```python
from build123d import *

# Parameters (mm, degrees)
F1_DEPTH = 40.7
F2_R     = 4
F3_DEPTH = 25


with BuildPart() as f1:
    # F0 (on Front) → F1 (new body)
    with BuildSketch(Plane.XZ):
        Polygon((7.9, 80), (0, 80), (0, 3), (3, 0), (80, 0), (80, 7.9), (7.9, 7.9), align=None)
    extrude(amount=F1_DEPTH)

    # F2 (on face) → F3 (cut)
    with BuildSketch(Plane.YZ.offset(7.9)):
        with Locations((-31.2, 59.8)):
            Circle(F2_R)
        with Locations((-31.2, 46.8)):
            Circle(F2_R)
        with Locations((-10.5, 46.8)):
            Circle(F2_R)
        with Locations((-10.5, 59.8)):
            Circle(F2_R)
    extrude(amount=-F3_DEPTH, mode=Mode.SUBTRACT)


solid = f1.part
```
Could you check a few things on this model? Use its own coordinates, in mm. A direction names the side the tool comes from. Round coordinates to 2 decimals unless told otherwise and drop trailing zeros. Loops run counter-clockwise (first coordinate to the right, second up) from the corner with the lowest first, then second, coordinate; pieces in that order, holes last. Notation, with made-up numbers: (52.5, -14.75) - (72.5, -14.75) arc R29 cw to (72.5, 12.25) - close; hole circle Ø7 at (35, -18). An arc over 180 degrees is marked (long way). Answer in a Markdown table with one row per item. Add a question column.
(1) I need wall thicknesses on line 1 along Z through (x, y) = (3.25, -31.2); line 2 along Y through (x, z) = (2, 46); line 3 along Z through (x, y) = (2, -31) (3 decimals). Which ranges of each line are inside material? Lowest first, please.
(2) If we section it at C-C (y = -16): Please give me the cut outline in (x, z).
(3) For faces 5 (the face through (0, -20, 42)), 6 (the face through (44, -20, 7.9)), which set-ups out of +Z, -Z, +X, -X, +Y, -Y let a thin tool reach every point of the face, with its end or its side?
(4) If we section it at B-B (z = 46.8): Please give me the cut outline in (x, y).
(5) If we mould it in two halves opening along Z, with no side actions, what happens to faces 1 (the face through (41, -20, 0)), 2 (the face through (7.9, -20, 43)), 3 (the face through (4.005, -11.367, 55.895)), 4 (the face through (4.005, -27.505, 58.268))? For each: pulls with the +Z half, pulls with the -Z half, needs draft (parallel to the pull), parting line crosses it, or undercut.
(6) If we section it at A-A (y = -31.2): Please give me the cut outline in (x, z).
(7) I'm going to push flat-ended pins straight in: pin 1 (8 mm diameter, centred on x = 23.5, y = -15.5, fed in from +Z); pin 2 (10.5 mm diameter, centred on y = -10.5, z = 59.8, fed in from -X); pin 3 (13 mm diameter, centred on y = -10.5, z = 46.8, fed in from +X). Where does each tip first touch, or does it pass through?
(8) If we section it at D-D (z = 62): Please give me the cut outline in (x, y).
Model answer:
| question | item | result |
|---|---|---|
| 1 | line 1 | z = 0 to 42.8, 50.8 to 55.8, 63.8 to 80 |
| 1 | line 2 | y = -40.7 to -35.12, -27.28 to -14.42, -6.58 to 0 |
| 1 | line 3 | z = 1 to 42.805, 50.795 to 55.805, 63.795 to 80 |
| 2 | outline | (0, 3) - (3, 0) - (80, 0) - (80, 7.9) - (7.9, 7.9) - (7.9, 80) - (0, 80) - close |
| 3 | face 5 | +Z, -Z, -X, +Y, -Y |
| 3 | face 6 | +Z, +X, +Y, -Y |
| 4 | outline | (0, -40.7) - (7.9, -40.7) - (7.9, -35.2) - (0, -35.2) - close; (0, -27.2) - (7.9, -27.2) - (7.9, -14.5) - (0, -14.5) - close; (0, -6.5) - (7.9, -6.5) - (7.9, 0) - (0, 0) - close |
| 5 | face 1 | pulls with the -Z half |
| 5 | face 2 | needs draft |
| 5 | face 3 | undercut |
| 5 | face 4 | undercut |
| 6 | outline | (0, 3) - (3, 0) - (80, 0) - (80, 7.9) - (7.9, 7.9) - (7.9, 42.8) - (0, 42.8) - close; (0, 50.8) - (7.9, 50.8) - (7.9, 55.8) - (0, 55.8) - close; (0, 63.8) - (7.9, 63.8) - (7.9, 80) - (0, 80) - close |
| 7 | pin 1 | stops at z = 7.9 |
| 7 | pin 2 | stops at x = 0 |
| 7 | pin 3 | stops at x = 7.9 |
| 8 | outline | (0, -40.7) - (7.9, -40.7) - (7.9, -34.54) - (0, -34.54) - close; (0, -27.86) - (7.9, -27.86) - (7.9, -13.84) - (0, -13.84) - close; (0, -7.16) - (7.9, -7.16) - (7.9, 0) - (0, 0) - close |
